Autodesk Inventor part; units mm, degrees
ref_plane "YZ Plane" through (0, 0, 0) normal (1, 0, 0) x (0, 1, 0)
ref_plane "XZ Plane" through (0, 0, 0) normal (0, 1, 0) x (-1, 0, 0)
ref_plane "XY Plane" through (0, 0, 0) normal (0, 0, 1) x (1, 0, 0)
sketch "スケッチ1" plane through (0, 0, 0) normal (0, 0, 1) x (1, 0, 0)
  circle A0 centre (0, 0) radius 13.5
  dimension "d0" = 27
extrude "押し出し1" add sketch "スケッチ1" along normal blind 3
sketch "スケッチ2" plane through (0, 0, 3) normal (0, 0, 1) x (1, 0, 0)
  point P0 (0, 0)
  point P1 (0, 10)
  point P2 (-8.6603, -5)
  point P3 (8.6603, -5)
  dimension "d3" = 10
  dimension "d6" = 360
hole "穴1" at (0, 10, 3) at (-8.6603, -5, 3) at (8.6603, -5, 3) direction (0, 0, -1) diameter 2.7 depth 3
sketch "スケッチ3" plane through (0, 0, 0) normal (0, 0, -1) x (-1, 0, 0)
  circle A0 centre (0, 0) radius 13.5
  line L0 (0, -13.5) -> (50, -13.5)
  line L1 (50, -13.5) -> (50, 13.5)
  line L2 (50, 13.5) -> (0, 13.5)
  line L3 (0, 13.5) -> (0, -13.5)
  line L4 (0, 0) -> (50, 0) construction
  line L5 (50, 13.5) -> (40, 13.5)
  line L6 (40, 13.5) -> (40, 22.15)
  line L7 (40, 22.15) -> (50, 22.15)
  line L8 (50, 22.15) -> (50, 13.5)
  line L9 (50, -13.5) -> (40, -13.5)
  line L10 (40, -13.5) -> (40, -14.85)
  line L11 (40, -14.85) -> (50, -14.85)
  line L12 (50, -14.85) -> (50, -13.5)
  point P0 (40, -13.5)
  dimension "d15" = 27
  dimension "d16" = 50
  dimension "d18" = 10
  dimension "d32" = 10
  dimension "d33" = 1.35
  dimension "d34" = 37
extrude "押し出し2" add sketch "スケッチ3" against normal up to surface (3 mm away) contours A0 L2 L1 L0 | L6 L7 L8 L2 | L0 L12 L11 L10
sketch "スケッチ4" plane through (0, 0, 0) normal (0, 0, -1) x (-1, 0, 0)
  line L0 (0, -13.5) -> (40, -13.5)
  line L1 (45, -13.5) -> (45, 22.15) construction
  line L2 (50, 22.15) -> (40, 22.15)
  line L3 (40, -14.85) -> (50, -14.85)
  line L4 (50, -14.85) -> (50, 22.15)
  point P0 (0, 0)
  point P1 (45, -9.85)
  point P2 (45, 17.15)
  dimension "d23" = 27
  dimension "d35" = 5
  dimension "d37" = 5
hole "穴2" at (-45, -9.85, 0) at (-45, 17.15, 0) direction (0, 0, 1) diameter 4.2 depth 3
fillet "フィレット1" radius 4 6 edges at (-40, 13.5, 1.5) (-40, 22.15, 1.5) (-50, 22.15, 1.5) (-50, -14.85, 1.5) (-40, -14.85, 1.5) (-40, -13.5, 1.5)
properties part number "finger2" material "アルミニウム 6061"
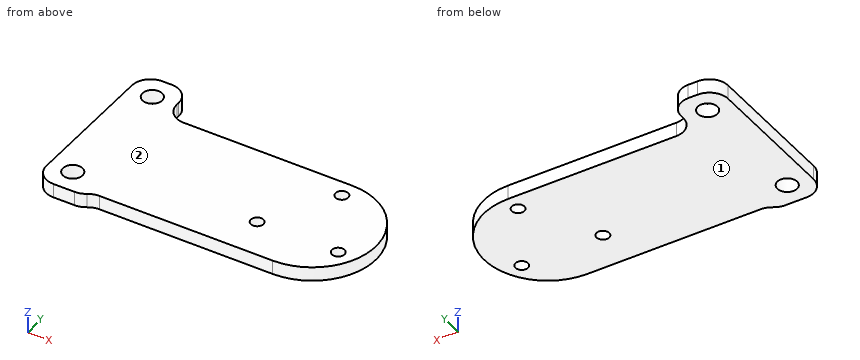
Model file for the job. Use its own axes, mm. Face numbers are marked on the shaded views. Round coordinates to 2 decimals unless told otherwise and drop trailing zeros. Write each loop counter-clockwise with the first axis right and the second up, starting at its lowest first coordinate (ties: lowest second). Pieces come first, ordered by that corner, then holes. Notation, with made-up numbers: (23.25, 58) - (51.25, 58) arc R10 cw to (51.25, 69) - close; hole circle Ø5 at (35.25, 18.5). An arc over 180 degrees is marked (long way). One line per item, written item: value.
(1) Cut at A-A, the plane y = -5.5. Give the cut face in (x, z), plus the area to 3 significant figures.
Values follow:
outline: (-50, 0) - (-9.91, 0) - (-9.91, 3) - (-50, 3) - close; (-7.41, 0) - (7.41, 0) - (7.41, 3) - (-7.41, 3) - close; (9.91, 0) - (12.33, 0) - (12.33, 3) - (9.91, 3) - close
area: 172 mm²
(2) Cut at B-B, the plane y = -9.85. Give the cut face in (x, z).
Values follow:
outline: (-50, 0) - (-47.1, 0) - (-47.1, 3) - (-50, 3) - close; (-42.9, 0) - (9.23, 0) - (9.23, 3) - (-42.9, 3) - close
(3) Drop flat-ended pins along their axis: P1, Ø1, axis at x = -2, z = 2.5, coming from the -Y side; P2, Ø1.5, axis at x = -26, z = 2, coming from the +Y side. Give the stop position or say it passes through.
Values follow:
P1: stops at y = -13.5
P2: stops at y = 13.5
(4) Two-plate mould, pull along Z, no slides. Class the marked faces 1 and 2: pulls with the +Z half, pulls with the -Z half, needs draft (parallel to the pull), parting line crosses it, or undercut.
Values follow:
face 1: pulls with the -Z half
face 2: pulls with the +Z half
(5) Wall check: probe 1 along Y at (x, z) = (-45, 1.25); probe 2 along X at (y, z) = (17.15, 1.8); probe 3 along X at (y, z) = (-5, 0.6). Give the ranges that are in metal, low to high.
Values follow:
probe 1: y = -14.85 to -11.95, -7.75 to 15.05, 19.25 to 22.15
probe 2: x = -50 to -47.1, -42.9 to -39.98
probe 3: x = -50 to -10.01, -7.31 to 7.31, 10.01 to 12.54
(6) Cut at D-D, the plane x = -3.5. Give the cut face in (y, z), plus the area to 3 significant figures.
Values follow:
outline: (-13.5, 0) - (13.5, 0) - (13.5, 3) - (-13.5, 3) - close
area: 81.0 mm²
(7) Cut at C-C, the plane z = 1.2. Give the cut face in (x, y) (3 decimals), plus the area to 3 significant figures.
Values follow:
outline: (-50, -10.85) arc R4 ccw to (-46, -14.85) - (-41.451, -14.85) arc R4 ccw to (-39.227, -14.175) arc R4 cw to (-37.004, -13.5) - (0, -13.5) arc R13.5 ccw to (0, 13.5) - (-36, 13.5) arc R4 cw to (-40, 17.5) - (-40, 18.15) arc R4 ccw to (-44, 22.15) - (-46, 22.15) arc R4 ccw to (-50, 18.15) - close; hole circle Ø4.2 at (-45, -9.85); hole circle Ø4.2 at (-45, 17.15); hole circle Ø2.7 at (-8.66, -5); hole circle Ø2.7 at (0, 10); hole circle Ø2.7 at (8.66, -5)
area: 1,690 mm²
